```python
from build123d import *

# Parameters (mm, degrees)
F0_W     = 25
F0_H     = 35
F1_DEPTH = 10
F2_SIZE2 = 34.99999
F2_SIZE  = 7.99999
F3_W     = 9
F3_H     = 28
F4_DEPTH = 33.35697
F5_W     = 10
F5_H     = 13
F6_DEPTH = 25


# Not quite as in the source:
# - a fillet or chamfer is up to 0.001 mm smaller than in the source, because OpenCascade refuses the exact size


with BuildPart() as f1:
    # F0 (on Front) → F1 (new body, symmetric)
    with BuildSketch(Plane.XZ):
        with Locations((-14.1274514172, 17.5)):
            Rectangle(F0_W, F0_H)
    extrude(amount=F1_DEPTH, both=True)

    # F2 (size 8 and 35 in the source; OpenCascade refuses exactly that, so slightly less here)
    f2_edges = [f1.edges().sort_by_distance(p)[0] for p in [
        (-1.627451, 0, 35),
    ]]
    f2_side = f1.faces().sort_by_distance((-14.127451, 0, 35))[0]
    chamfer(f2_edges, length=F2_SIZE, length2=F2_SIZE2, reference=f2_side)

    # F3 (on face) → F4 (cut)
    with BuildSketch(Plane(origin=(0, 10, 0), x_dir=(-1, 0, 0), z_dir=(0, 1, 0))):
        with Locations((18.1274514172, 17.5)):
            Rectangle(F3_W, F3_H)
    extrude(amount=-F4_DEPTH, mode=Mode.SUBTRACT)

    # F5 (on face) → F6 (cut)
    with BuildSketch(Plane(origin=(-26.6274514172, 0, 0), x_dir=(0, -1, 0), z_dir=(-1, 0, 0))):
        with BuildLine():
            ThreePointArc((5, 24), (0, 29), (-5, 24))
            Line((-5, 24), (5, 24))
        make_face()
        with Locations((0, 17.5)):
            Rectangle(F5_W, F5_H)
        with BuildLine():
            Line((5, 11), (-5, 11))
            ThreePointArc((-5, 11), (0, 6), (5, 11))
        make_face()
    extrude(amount=-F6_DEPTH, mode=Mode.SUBTRACT)


solid = f1.part
```
The listing builds one solid part. Answer for the finished solid, in the listing's coordinates (mm). A direction names the side the tool comes from. Coordinates: 2 decimals unless noted, no trailing zeros. Order: outer loops, then holes, each group sorted by start corner. A loop starts at its lowest first (then second) coordinate and runs counter-clockwise, first axis right, second up. Notation, with made-up numbers: M 69,51.25 L 118,51.25 A33 ccw 118,81.25 Z; hole C -10,50 d5. An arc over 180 degrees is marked long. Answer as a JSON object with one key per item and string values. Group by question number.
1. A flat-ended cylindrical pin translates along its axis: P1, Ø1.5, axis at y = 4, z = 26.5, coming from the +X side. Find the tip coordinate at first contact, or state that the pin passes through.
2. Section D-D on z = 17 is taken. Write down the section's boundary in (x, y).
3. Section A-A on x = -20 is taken. Write down the section's boundary in (y, z).
4. Determine the mould class of faces 4 (the flat face through (-25, -5, 17)), 5 (the flat face through (-12, -10, 18)), 6 (the flat face through (-26.627, -7, 17)) for opening direction Y: released by +Y, released by -Y, zero draft, split by the parting line, or undercut.
5. Straight lines are drawn through the part: line 1 (Z direction, x = -19.25, y = 6.5); line 2 (Y direction, x = -7.5, z = 14.5); line 3 (X direction, y = 9, z = 18). For each, find the intervals that lie inside material, in ascending order.
6. A tool of negligible diameter and unlimited length cuts with its end or side. For faces 1 (the flat face through (-10, 5, 17)), 2 (the flat face through (-22.627, 7, 17)), 3 (the flat face through (-18, 0, 35)), from which of +Z, -Z, +X, -X, +Y, -Y can it reach the whole face along a straight path? Write none if from no direction.
Values follow:
{
 "1": {"P1": "x = -7.57"},
 "2": {"outline": "M -26.63,-10 L -22.63,-10 L -22.63,-5 L -26.63,-5 Z; M -26.63,5 L -22.63,5 L -22.63,10 L -26.63,10 Z; M -13.63,-10 L -5.51,-10 L -5.51,-5 L -13.63,-5 Z; M -13.63,5 L -5.51,5 L -5.51,10 L -13.63,10 Z"},
 "3": {"outline": "M -10,0 L 10,0 L 10,3.5 L -10,3.5 Z; M -10,31.5 L 10,31.5 L 10,35 L -10,35 Z"},
 "4": {"face 4": "undercut", "face 5": "released by -Y", "face 6": "zero draft"},
 "5": {"line 1": "0 to 3.5, 31.5 to 35", "line 2": "-10 to -5, 5 to 10", "line 3": "-26.63 to -22.63, -13.63 to -5.74"},
 "6": {"face 1": "+X, -X", "face 2": "+Y, -Y", "face 3": "+Z, +X, -X, +Y, -Y"}
}
